from build123d import *

# Parameters (mm, degrees)
EXTRUDE_1_DEPTH        = 1056
HOLE_WIZARD_7_0_7_1_D  = 7
CUT_EXTRUDE_2_REACH    = 1059.571
SKETCH_5_R             = 6
HOLE_WIZARD_M5_1_D     = 5
HOLE_WIZARD_M5_1_DEPTH = 4.5
HOLE_WIZARD_M5_2_D     = 5
HOLE_WIZARD_M5_2_DEPTH = 4.5
CUT_EXTRUDE_3_DEPTH    = 1058.795821508


with BuildPart() as part:
    # 草图1 → 凸台-拉伸1 (new body)
    with BuildSketch(Plane.XY):
        Polygon((36, -0.5), (36, -7.842615501), (10, -45), (0, -45), (0, 0), (0, 5), (4, 5), (4, -0.5), (7, -0.5), (7, 0), (17, 0), (17, -0.5), (23, -0.5), (23, 0), (33, 0), (33, -0.5), align=None)
        with BuildLine():
            Line((33, -5), (33, -6.582130473))
            ThreePointArc((33, -6.582130473), (32.953765498, -6.882682255), (32.819337252, -7.155442314))
            Line((32.819337252, -7.155442314), (8.736247988, -41.573311842))
            ThreePointArc((8.736247988, -41.573311842), (8.378802584, -41.886936255), (7.916910736, -42))
            Line((7.916910736, -42), (5.5, -42))
            ThreePointArc((5.5, -42), (4.792893219, -41.707106781), (4.5, -41))
            Line((4.5, -41), (4.5, -5))
            ThreePointArc((4.5, -5), (4.792893219, -4.292893219), (5.5, -4))
            Line((5.5, -4), (32, -4))
            ThreePointArc((32, -4), (32.707106781, -4.292893219), (33, -5))
        make_face(mode=Mode.SUBTRACT)
    extrude(amount=EXTRUDE_1_DEPTH)

    # Ø7.0 (7) 直径孔1 (through all)
    with Locations(Plane.ZY):
        with Locations((68.68, -22), (874, -22)):
            Hole(HOLE_WIZARD_7_0_7_1_D / 2)

    # 切除-拉伸2: up to this plane
    cut_extrude_2_end = Plane(origin=(32.819337252, -7.155442314, 1056), z_dir=(-0.8193372517042258, 0.5733118418188885, 0))
    # 草图5 → 切除-拉伸2 (cut, up to the surface)
    with BuildSketch(Plane(origin=(36, 0, 0), x_dir=(0, 0, -1), z_dir=(1, 0, 0)), mode=Mode.PRIVATE) as cut_extrude_2_sk1:
        with Locations(Location((-68.68, -22.072492254, 0), (0, 0, 90))):
            Circle(SKETCH_5_R)
    cut_extrude_2_tool1 = split(extrude(cut_extrude_2_sk1.sketch, amount=-CUT_EXTRUDE_2_REACH, mode=Mode.PRIVATE), bisect_by=cut_extrude_2_end, keep=Keep.BOTH, mode=Mode.PRIVATE)
    add(cut_extrude_2_tool1.solids().sort_by_distance((36, -22.072492, 68.68))[0], mode=Mode.SUBTRACT)
    # 草图5 → 切除-拉伸2 (cut, up to the surface)
    with BuildSketch(Plane(origin=(36, 0, 0), x_dir=(0, 0, -1), z_dir=(1, 0, 0)), mode=Mode.PRIVATE) as cut_extrude_2_sk2:
        with Locations(Location((-874, -22, 0), (0, 0, 90))):
            Circle(SKETCH_5_R)
    cut_extrude_2_tool2 = split(extrude(cut_extrude_2_sk2.sketch, amount=-CUT_EXTRUDE_2_REACH, mode=Mode.PRIVATE), bisect_by=cut_extrude_2_end, keep=Keep.BOTH, mode=Mode.PRIVATE)
    add(cut_extrude_2_tool2.solids().sort_by_distance((36, -22, 874))[0], mode=Mode.SUBTRACT)

    # M5 螺纹孔1
    with Locations(Plane.ZY):
        with Locations((18.636598419, -11.935996902), (18.636598419, -32), (118.675555099, -11.935996902), (118.675555099, -32)):
            Hole(HOLE_WIZARD_M5_1_D / 2, depth=HOLE_WIZARD_M5_1_DEPTH)

    # M5 螺纹孔2
    with Locations(Plane.ZY):
        with Locations((850, -12), (898, -12), (898, -32), (850, -32)):
            Hole(HOLE_WIZARD_M5_2_D / 2, depth=HOLE_WIZARD_M5_2_DEPTH)

    # 草图11 → 切除-拉伸3 (cut, through all)
    with BuildSketch(Plane(origin=(0, 5, 0), x_dir=(1, 0, 0), z_dir=(0, 1, 0))):
        Polygon((36, -1056), (0, -1040.940873789), (0, -1056), align=None)
    extrude(amount=-CUT_EXTRUDE_3_DEPTH, mode=Mode.SUBTRACT)


solid = part.part
Here's how the part is built. I have some questions about the finished solid (model axes, mm). A direction names the side the tool comes from. Round coordinates to 2 decimals unless told otherwise and drop trailing zeros. Loops run counter-clockwise (first coordinate to the right, second up) from the corner with the lowest first, then second, coordinate; pieces in that order, holes last. Notation, with made-up numbers: (45.5, 89) - (103.5, 89) arc R36 cw to (103.5, 123) - close; hole circle Ø4 at (79, -1.5). An arc over 180 degrees is marked (long way). One line per question, with ' | ' between items. Start each with the question number.
Q1. Please list where these lines run through material, in increasing order: line 1 (Y direction, x = 3, z = 850); line 2 (Y direction, x = 1, z = 68); line 3 (X direction, y = -6.5, z = 303). Write a range as [from, to].
Q2. For faces 4 (the flat face through (19, -4, 520)), 5 (the flat face through (3.42, -18.03, 1042.37)), which set-ups out of +Z, -Z, +X, -X, +Y, -Y let a thin tool reach every point of the face, with its end or its side?
Q3. We'd pull the mould along X, two halves only. Please class faces 1 (the flat face through (0, -20, 513)), 2 (the flat face through (23.182, -26.161, 520.608)), 3 (the flat face through (4.5, -23, 514)): +X half, -X half, draft (parallel to the pull), parting line (faces both ways), or undercut.
Q4. I want a section at A-A (z = 369). Write out the boundary of the cut face in (x, y).
Q5. Will these pins go through, and if not, where does the flat tip stop? pin 1 (4.5 mm diameter, centred on y = -32, z = 118.68, fed in from +X); pin 2 (3.5 mm diameter, centred on x = 34.5, z = 310, fed in from +Y); pin 3 (1.5 mm diameter, centred on y = -13, z = 781.5, fed in from +X).
Response values:
1) line 1: y = [-45, -34.5], [-29.5, -14.5], [-9.5, 5] | line 2: y = [-45, -25.43], [-18.57, 5] | line 3: x = [0, 4.5], [33, 36]
2) face 4: +Z, -Z | face 5: +Z, -X, +Y, -Y
3) face 1: -X half | face 2: +X half | face 3: undercut
4) outline: (0, -45) - (10, -45) - (36, -7.84) - (36, -0.5) - (33, -0.5) - (33, 0) - (23, 0) - (23, -0.5) - (17, -0.5) - (17, 0) - (7, 0) - (7, -0.5) - (4, -0.5) - (4, 5) - (0, 5) - close; hole (4.5, -41) arc R1 ccw to (5.5, -42) - (7.92, -42) arc R1 ccw to (8.74, -41.57) - (32.82, -7.16) arc R1 ccw to (33, -6.58) - (33, -5) arc R1 ccw to (32, -4) - (5.5, -4) arc R1 ccw to (4.5, -5) - close
5) pin 1: stops at x = 20.67 | pin 2: stops at y = 0 | pin 3: stops at x = 32.92
